from build123d import *

# Parameters (mm, degrees)
F0_W      = 38.1
F0_H      = 38.1
F1_DEPTH  = 0.79375
F2_W      = 38.1
F2_H      = 38.1
F2_W_2    = 34.925
F2_H_2    = 34.925
F3_DEPTH  = 6.35
F4_W      = 1.27
F4_H      = 29.845
F4_W_2    = 10.795
F4_H_2    = 1.27
F5_DEPTH  = 4.445
F6_W      = 10.795
F6_H      = 1.27
F7_DEPTH  = 4.445
F8_R      = 1.27
F9_DEPTH  = 0.396875
F10_R     = 1.27
F11_DEPTH = 0.396875
F12_DEPTH = 0.396875


with BuildPart() as f1:
    # F0 (on Top) → F1 (new body)
    with BuildSketch(Plane.XY):
        with Locations((0.218246, 6.881682)):
            Rectangle(F0_W, F0_H)
    extrude(amount=F1_DEPTH)

    # F2 (on face) → F3 (join)
    with BuildSketch(Plane.XY.offset(0.79375)):
        with Locations((0.218246, 6.881682)):
            Rectangle(F2_W, F2_H)
        with Locations((0.218246, 6.881682)):
            Rectangle(F2_W_2, F2_H_2, mode=Mode.SUBTRACT)
    extrude(amount=F3_DEPTH)

    # F4 (on face) → F5 (join)
    with BuildSketch(Plane.XY.offset(0.79375)):
        with Locations((-11.529254, 4.341682)):
            Rectangle(F4_W, F4_H)
        with Locations((-5.179254, 9.421682)):
            Rectangle(F4_W, F4_H)
        with Locations((1.170746, 4.341682)):
            Rectangle(F4_W, F4_H)
        with Locations((12.283246, 12.279182)):
            Rectangle(F4_W_2, F4_H_2)
        with Locations((12.283246, 18.629182)):
            Rectangle(F4_W_2, F4_H_2)
    extrude(amount=F5_DEPTH)

    # F6 (on face) → F7 (join)
    with BuildSketch(Plane.XY.offset(0.79375)):
        with Locations((12.283246, 5.929182)):
            Rectangle(F6_W, F6_H)
    extrude(amount=F7_DEPTH)

    # F8 (on face) → F9 (cut)
    with BuildSketch(Plane.XY.offset(0.79375)):
        with Locations((-14.704254, -6.816329)):
            Circle(F8_R)
    extrude(amount=F9_DEPTH, mode=Mode.SUBTRACT)

    # F10 (on face) → F11 (cut)
    with BuildSketch(Plane.XY.offset(0.79375)):
        with Locations((15.417561, 9.104182)):
            Circle(F10_R)
    extrude(amount=-F11_DEPTH, mode=Mode.SUBTRACT)

    # F8 (on face) → F12 (cut)
    with BuildSketch(Plane.XY.offset(0.79375)):
        with Locations((-14.704254, -6.816329)):
            Circle(F8_R)
    extrude(amount=-F12_DEPTH, mode=Mode.SUBTRACT)


solid = f1.part
Build history of the part. All positions in model axes, mm. A direction names the side the tool comes from. Coordinates: 2 decimals unless noted, no trailing zeros. Order: outer loops, then holes, each group sorted by start corner. A loop starts at its lowest first (then second) coordinate and runs counter-clockwise, first axis right, second up. Notation, with made-up numbers: (-5, 52.5) - (28, 52.5) arc R28 cw to (28, 90.5) - close; hole circle Ø10 at (33.25, 37.25). An arc over 180 degrees is marked (long way). Put each result on its own line as item: value.
1. Pull direction X, two halves, no side cores. Call faces 1 (the face through (15, 9, 0.397)), 2 (the face through (19.268, 7, 4)), 3 (the face through (0, -12.168, 4)): pulls with the +X half, pulls with the -X half, needs draft (parallel to the pull), parting line crosses it, or undercut.
Answer sheet:
face 1: undercut
face 2: pulls with the +X half
face 3: needs draft
2. Tool access for faces 4 (the face through (1, 19.264, 3)), 5 (the face through (0, 25.932, 4)): list every direction of +Z, -Z, +X, -X, +Y, -Y with a clear straight run to the whole face (end or side of a thin tool).
Answer sheet:
face 4: +Z
face 5: +Z, -Z, +X, -X, +Y
3. Saw through at C-C (y = 15.5). Write the cut outline in (x, z), and give its area (3 significant figures).
Answer sheet:
outline: (-18.83, 0) - (19.27, 0) - (19.27, 7.14) - (17.68, 7.14) - (17.68, 0.79) - (1.81, 0.79) - (1.81, 5.24) - (0.54, 5.24) - (0.54, 0.79) - (-4.54, 0.79) - (-4.54, 5.24) - (-5.81, 5.24) - (-5.81, 0.79) - (-10.89, 0.79) - (-10.89, 5.24) - (-12.16, 5.24) - (-12.16, 0.79) - (-17.24, 0.79) - (-17.24, 7.14) - (-18.83, 7.14) - close
area: 67.3 mm^2
4. Drop a flat-ended pin along its axis: P1, Ø8, axis at x = 5.5, y = 10, coming from the +Z side. Give the stop position or say it passes through.
Answer sheet:
P1: stops at z = 5.24
5. Probe line 1 along X through (y, z) = (17, 1.25); line 2 along Y through (x, z) = (17.5, 4.5); line 3 along X through (y, z) = (24, 1.5). List the from-to ranges inside material, lowest first. Write a range as [from, to].
Answer sheet:
line 1: x = [-18.83, -17.24], [-12.16, -10.89], [-5.81, -4.54], [0.54, 1.81], [17.68, 19.27]
line 2: y = [-12.17, -10.58], [5.29, 6.56], [11.64, 12.91], [17.99, 19.26], [24.34, 25.93]
line 3: x = [-18.83, -17.24], [-5.81, -4.54], [17.68, 19.27]
6. Saw through at D-D (x = 4.5). Write the cut outline in (y, z), and give its area (3 significant figures).
Answer sheet:
outline: (-12.17, 0) - (25.93, 0) - (25.93, 7.14) - (24.34, 7.14) - (24.34, 0.79) - (-10.58, 0.79) - (-10.58, 7.14) - (-12.17, 7.14) - close
area: 50.4 mm^2
7. Saw through at A-A (x = 8.5). Write the cut outline in (y, z).
Answer sheet:
outline: (-12.17, 0) - (25.93, 0) - (25.93, 7.14) - (24.34, 7.14) - (24.34, 0.79) - (19.26, 0.79) - (19.26, 5.24) - (17.99, 5.24) - (17.99, 0.79) - (12.91, 0.79) - (12.91, 5.24) - (11.64, 5.24) - (11.64, 0.79) - (6.56, 0.79) - (6.56, 5.24) - (5.29, 5.24) - (5.29, 0.79) - (-10.58, 0.79) - (-10.58, 7.14) - (-12.17, 7.14) - close
